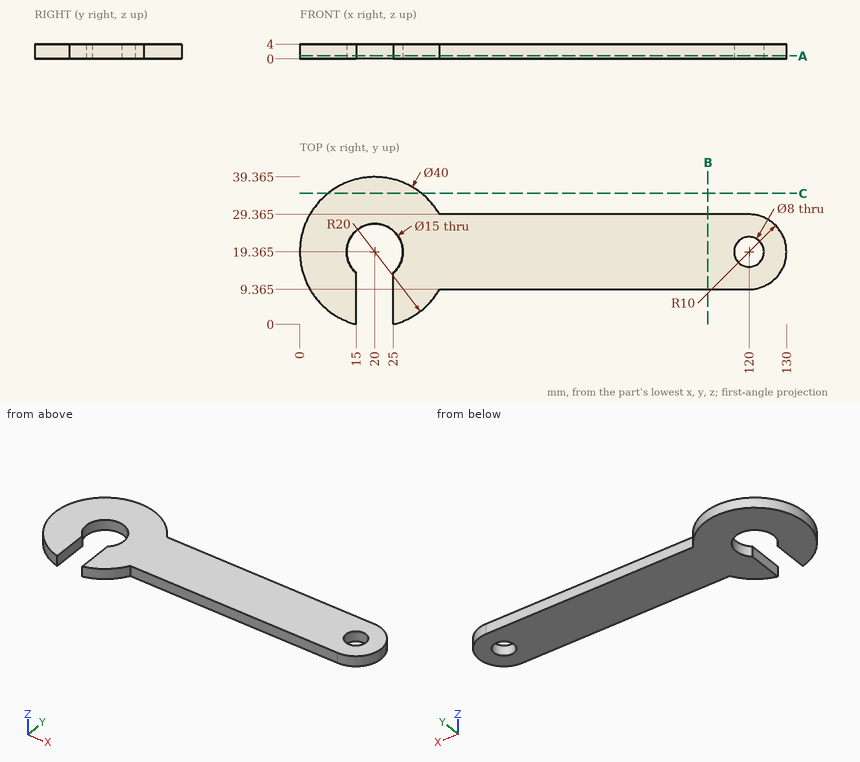
Source: three-view drawing plus pictorial views. Frame: mm from the lowest corner of the part. Round coordinates to 2 decimals unless told otherwise and drop trailing zeros. Order: outer loops, then holes, each group sorted by start corner. A loop starts at its lowest first (then second) coordinate and runs counter-clockwise, first axis right, second up. Notation, with made-up numbers: (35.5, -12.75) -> (82.5, -12.75) arc R7 ccw to (82.5, -2.75) -> close; hole circle Ø6 at (89.5, 68.5). An arc over 180 degrees is marked (long way). Use one line per item in the form item = value. Start each with the question number.
1. Cut plane A-A (z = 0.8). Return the cut outline in (x, y) (1 decimal).
2. Cut plane B-B (x = 109). Return the cut outline in (y, z) (3 decimals).
3. Line query: probe 1 along Y at (x, z) = (120, 1.5) (3 decimals); probe 2 along X at (y, z) = (20.5, 2.5); probe 3 along Y at (x, z) = (20, 3.1) (3 decimals). Output: solid intervals per line, ascending.
4. Cut plane C-C (y = 35). Return the cut outline in (x, z), then the cut area to 3 significant figures.
5. Pin query (flat end, axial travel): pin 1 Ø1 at (x, z) = (107, 0.5) entering from -Y (3 decimals); pin 2 Ø1 at (y, z) = (11.5, 3) entering from -X; pin 3 Ø1.2 at (y, z) = (9.5, 2) entering from -X. Return the tip coordinate at first contact, or that it passes through.
Solution:
q1.outline = (15, 0) -> (15, 13.8) arc R7.5 cw (long way) to (25, 13.8) -> (25, 0) arc R20 ccw to (37.3, 9.4) -> (120, 9.4) arc R10 ccw to (120, 29.4) -> (37.3, 29.4) arc R20 ccw (long way) to start; hole circle Ø8 at (120, 19.4)
q2.outline = (9.365, 0) -> (29.365, 0) -> (29.365, 4) -> (9.365, 4) -> close
q3.probe_1 = 9.365 to 15.365, 23.365 to 29.365
q3.probe_2 = 0.03 to 12.59, 27.41 to 116.16, 123.84 to 129.94
q3.probe_3 = 26.865 to 39.365
q4.outline = (7.53, 0) -> (32.47, 0) -> (32.47, 4) -> (7.53, 4) -> close
q4.area = 99.8 mm^2
q5.pin_1 = 9.365
q5.pin_2 = 1.41
q5.pin_3 = 2.28
